For this review, take the finished solid that the model builds, in its own axes (mm). Give positions to 0.01 mm unless a question says otherwise; leave off trailing zeros. Order: outer loops, then holes, each group sorted by start corner. A loop starts at its lowest first (then second) coordinate and runs counter-clockwise, first axis right, second up. Notation, with made-up numbers: (44, 63.5) - (48, 63.5) arc R19 cw to (48, 99.5) - close; hole circle Ø1 at (58.25, 73.25). An arc over 180 degrees is marked (long way). Use a Markdown table: item, result. Add a question column.
1) Wall thickness on L1, parallel to X at y = 15.2, z = 3.5; L2, parallel to X at y = -15.2, z = 3.25: over which ranges is each line inside the solid? List them lowest first.
2) We need section A-A on y = 15.2. Write out the cut boundary in (x, z).
3) Clearance check with flat-ended pins moving along their axes: P1, Ø2, axis at x = 6, z = 4.5, coming from the +Y side; P2, Ø3, axis at x = -15.2, y = 15.2, coming from the +Z side; P3, Ø0.8, axis at x = -2, z = 7, coming from the +Y side; P4, Ø1.5, axis at x = 5, y = 6, coming from the -Z side. State where each tip first meets the part, or that it passes through.
4) We need section D-D on x = -8.5. Write out the cut boundary in (y, z), then the cut area to 3 significant figures.
5) We need section C-C on z = 1.25. Write out the cut boundary in (x, y).
```python
from build123d import *

# Parameters (mm, degrees)
F0_W     = 33
F0_H     = 33
F1_DEPTH = 9
F2_W     = 3
F2_H     = 0.9
F2_W_2   = 7
F2_H_2   = 7.583788
F3_DEPTH = 3
F4_R     = 5
F5_DEPTH = 2
F6_R     = 1
F7_DEPTH = 25


with BuildPart() as f1:
    # F0 (on Top) → F1 (new body)
    with BuildSketch(Plane.XY):
        Rectangle(F0_W, F0_H)
    extrude(amount=F1_DEPTH)

    # F2 (on face) → F3 (join)
    with BuildSketch(Plane.XY.offset(9)):
        Polygon((-7.5, 16.6), (-7.5, 16.5), (-1.5, 16.5), (-1.5, 16.6), (-3, 16.6), (-6, 16.6), align=None)
        with Locations((-4.5, 17.05)):
            Rectangle(F2_W, F2_H)
        with Locations((2, -13.708106)):
            Rectangle(F2_W_2, F2_H_2)
    extrude(amount=-F3_DEPTH)

    # F4 (on face) → F5 (join)
    with BuildSketch(Plane(origin=(0, 0, 0), x_dir=(1, 0, 0), z_dir=(0, 0, -1))):
        with Locations((-8.5, -3.5)):
            Circle(F4_R)
    extrude(amount=F5_DEPTH)

    # F6 (on face) → F7 (cut)
    with BuildSketch(Plane(origin=(0, 0, 0), x_dir=(1, 0, 0), z_dir=(0, 0, -1))):
        with Locations((-15.2, -15.2)):
            Circle(F6_R)
        with Locations((15.2, 15.2)):
            Circle(F6_R)
    extrude(amount=-F7_DEPTH, mode=Mode.SUBTRACT)


solid = f1.part
```
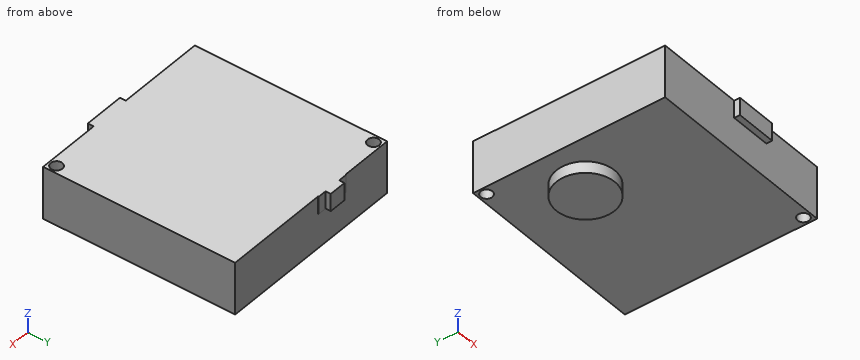
Checked values:
| question | item | result |
|---|---|---|
| 1 | L1 | -16.5 to -16.2, -14.2 to 16.5 |
| 1 | L2 | -16.5 to 14.2, 16.2 to 16.5 |
| 2 | outline | (-16.5, 0) - (-16.2, 0) - (-16.2, 9) - (-16.5, 9) - close; (-14.2, 0) - (16.5, 0) - (16.5, 9) - (-14.2, 9) - close |
| 3 | P1 | y = 16.5 |
| 3 | P2 | z = 9 |
| 3 | P3 | y = 16.6 |
| 3 | P4 | z = 0 |
| 4 | outline | (-16.5, 0) - (-1.5, 0) - (-1.5, -2) - (8.5, -2) - (8.5, 0) - (16.5, 0) - (16.5, 9) - (-16.5, 9) - close |
| 4 | area | 317 mm² |
| 5 | outline | (-16.5, -16.5) - (16.5, -16.5) - (16.5, 16.5) - (-16.5, 16.5) - close; hole circle Ø2 at (-15.2, 15.2); hole circle Ø2 at (15.2, -15.2) |
